Read the model definition and answer for the solid it produces. Units are mm, in the model's axes. A direction names the side the tool comes from. Coordinates: 2 decimals unless noted, no trailing zeros. Write each loop counter-clockwise with the first axis right and the second up, starting at its lowest first coordinate (ties: lowest second). Pieces come first, ordered by that corner, then holes.
Item 1: Determine the mould class of faces 1 (the face through (9.633, -0.338, 2.578)), 2 (the face through (0, 0, 3)), 3 (the face through (18.528, 6.466, -2.681)) for opening direction Y: released by +Y, released by -Y, zero draft, split by the parting line, or undercut.
Item 2: Section C-C (x = 16.75) is taken. Give the vertices of the cut face in (y, z).
Item 3: Section A-A (z = 0) is taken. Give the vertices of the cut face in (x, y).
Item 4: Section D-D (x = 12.5) is taken. Give the vertices of the cut face in (y, z).
Item 5: Straight lines are drawn through the part: probe 1 along Z at (x, y) = (7.5, 0); probe 2 along X at (y, z) = (4.5, 4.25); probe 3 along Z at (x, y) = (12.5, 0). For each, find the intervals that lie inside material, in ascending order.
Item 6: A tool of negligible diameter and unlimited length cuts with its end or side. For faces 4 (the face through (17.568, -6, 0)), 5 (the face through (19, 0, -3)), from which of +Z, -Z, +X, -X, +Y, -Y can it reach the whole face along a straight path? Write none if from no direction.
Item 7: Each of these flat-tipped pins is pushed along its axis until it touches: P1, Ø8, axis at x = 6, z = 2.5, coming from the -Y side; P2, Ø2, axis at x = 16.5, z = 3.5, coming from the -Y side; P3, Ø1, axis at x = 16, y = -4, coming from the +Z side. Where does it stop, or does it pass through?
from build123d import *

# Parameters (mm, degrees)
F2_R = 1
F3_R = 0.5


with BuildPart() as f1:
    # F0 (on Top) → F1 (revolve)
    with BuildSketch(Plane.XY):
        Polygon((12.8682, 3.5), (0, 3.5), (0, 2.6), (1.560832, 2.6), (17.439168, 2.6), (19, 2.6), (19, 7), (17.5682, 7), (17.5682, 5.8), (12.8682, 5.8), align=None)
    revolve(axis=Axis((8.987734, 0, 0), (1, 0, 0)))

    # F2
    f2_edges = [f1.edges().sort_by_distance(p)[0] for p in [
        (12.8682, -3.5, 0),
    ]]
    fillet(f2_edges, radius=F2_R)

    # F3
    f3_edges = [f1.edges().sort_by_distance(p)[0] for p in [
        (17.5682, -7, 0),
        (12.8682, -5.8, 0),
    ]]
    fillet(f3_edges, radius=F3_R)


solid = f1.part
Established:
1. face 1: undercut
1. face 2: zero draft
1. face 3: split by the parting line
2. outline: circle Ø11.6 at (0, 0); hole circle Ø5.2 at (0, 0)
3. outline: (0, -3.5) - (11.87, -3.5) arc R1 cw to (12.87, -4.5) - (12.87, -5.3) arc R0.5 ccw to (13.37, -5.8) - (17.57, -5.8) - (17.57, -6.5) arc R0.5 ccw to (18.07, -7) - (19, -7) - (19, -2.6) - (0, -2.6) - close; (0, 2.6) - (19, 2.6) - (19, 7) - (18.07, 7) arc R0.5 ccw to (17.57, 6.5) - (17.57, 5.8) - (13.37, 5.8) arc R0.5 ccw to (12.87, 5.3) - (12.87, 4.5) arc R1 cw to (11.87, 3.5) - (0, 3.5) - close
4. outline: circle Ø7.45 at (0, 0); hole circle Ø5.2 at (0, 0)
5. probe 1: z = -3.5 to -2.6, 2.6 to 3.5
5. probe 2: x = 17.57 to 19
5. probe 3: z = -3.72 to -2.6, 2.6 to 3.72
6. face 4: -X
6. face 5: +Z, -Z, +X, +Y, -Y
7. P1: stops at y = -3.5
7. P2: stops at y = -5.23
7. P3: stops at z = 4.62
